The figure shows three views and two pictorial views of one solid part (mm, origin at its lowest corner). Answer the questions. A direction names the side the tool comes from. Round coordinates to 2 decimals unless told otherwise and drop trailing zeros. Order: outer loops, then holes, each group sorted by start corner. A loop starts at its lowest first (then second) coordinate and runs counter-clockwise, first axis right, second up. Notation, with made-up numbers: (-10.75, -39) - (22.25, -39) arc R26 ccw to (22.25, -18) - close; hole circle Ø6 at (17, 88). An arc over 180 degrees is marked (long way). Answer in a Markdown table with one row per item.
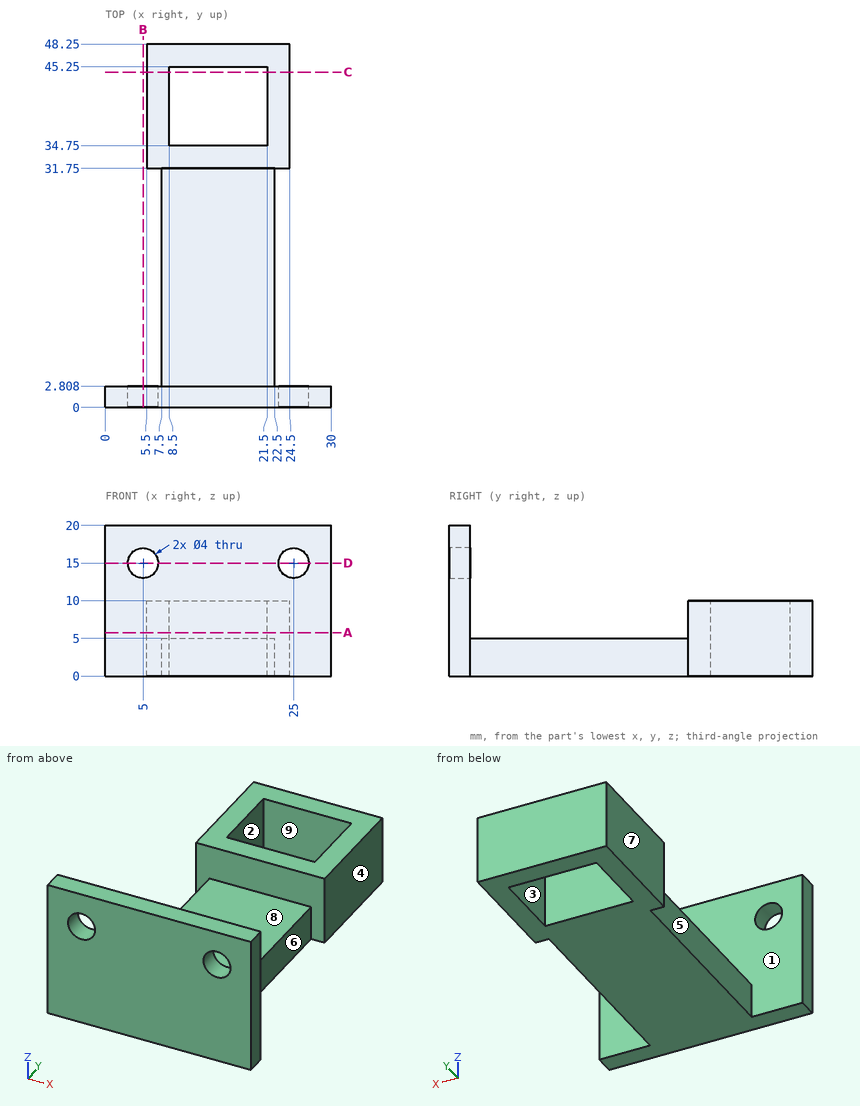
1) Which of the six approach directions +Z, -Z, +X, -X, +Y, -Y give full straight-line access (tool end or side, diameter ignored) to the marked faces 5, 6, 7, 8 and 9?
Filled in:
| item | result |
|---|---|
| face 5 | +Z, -Z, -X |
| face 6 | +Z, -Z, +X |
| face 7 | +Z, -Z, -X, +Y |
| face 8 | +Z, +X, -X |
| face 9 | +Z, -Z |
2) Find section C-C, the plane y = 44.5. Give the vertices of the cut face in (x, z), then the cut area to 3 significant figures.
Filled in:
| item | result |
|---|---|
| outline | (5.5, 0) - (8.5, 0) - (8.5, 10) - (5.5, 10) - close; (21.5, 0) - (24.5, 0) - (24.5, 10) - (21.5, 10) - close |
| area | 60.0 mm^2 |
3) Each of these flat-tipped pins is pushed along its axis until it touches: pin 1 (4 mm diameter, centred on y = 14, z = 2, fed in from +X); pin 2 (1 mm diameter, centred on x = 3.5, y = 36.5, fed in from -Z); pin 3 (5.5 mm diameter, centred on y = 22, z = 2.5, fed in from -X); pin 4 (5 mm diameter, centred on y = 41, z = 3.5, fed in from -X). Where does it stop, or does it pass through?
Filled in:
| item | result |
|---|---|
| pin 1 | stops at x = 22.5 |
| pin 2 | passes through |
| pin 3 | stops at x = 7.5 |
| pin 4 | stops at x = 5.5 |
4) Find the intervals of material crossed by probe 1 along X at (y, z) = (1.6, 15); probe 2 along Y at (x, z) = (5.75, 4.5); probe 3 along Z at (x, y) = (7, 43.5), in increasing order. Write a range as from..to.
Filled in:
| item | result |
|---|---|
| probe 1 | x = 0..3, 7..23, 27..30 |
| probe 2 | y = 0..2.81, 31.75..48.25 |
| probe 3 | z = 0..10 |
5) Find section B-B, the plane x = 5. Give the vertices of the cut face in (y, z).
Filled in:
| item | result |
|---|---|
| outline | (0, 0) - (2.81, 0) - (2.81, 13) - (0, 13) - close; (0, 17) - (2.81, 17) - (2.81, 20) - (0, 20) - close |
6) Find section A-A, the plane z = 5.75. Give the vertices of the cut face in (x, y), then the cut area to 3 significant figures.
Filled in:
| item | result |
|---|---|
| outline | (0, 0) - (30, 0) - (30, 2.81) - (0, 2.81) - close; (5.5, 31.75) - (24.5, 31.75) - (24.5, 48.25) - (5.5, 48.25) - close; hole (8.5, 34.75) - (21.5, 34.75) - (21.5, 45.25) - (8.5, 45.25) - close |
| area | 261 mm^2 |
7) The mould has two halves that part along X. Classify the marked faces 1, 2, 3 and 4: released by +X, released by -X, zero draft, split by the parting line, or undercut.
Filled in:
| item | result |
|---|---|
| face 1 | zero draft |
| face 2 | undercut |
| face 3 | undercut |
| face 4 | released by +X |
8) Find section D-D, the plane z = 15. Give the vertices of the cut face in (x, y).
Filled in:
| item | result |
|---|---|
| outline | (0, 0) - (3, 0) - (3, 2.81) - (0, 2.81) - close; (7, 0) - (23, 0) - (23, 2.81) - (7, 2.81) - close; (27, 0) - (30, 0) - (30, 2.81) - (27, 2.81) - close |
